Could you check a few things on this model? Use its own coordinates, in mm. A direction names the side the tool comes from. Round coordinates to 2 decimals unless told otherwise and drop trailing zeros. Write each loop counter-clockwise with the first axis right and the second up, starting at its lowest first coordinate (ties: lowest second). Pieces come first, ordered by that corner, then holes. Notation, with made-up numbers: (4, 27) -> (15, 27) arc R15 ccw to (15, 43) -> close; hole circle Ø7 at (58, -22). An arc over 180 degrees is marked (long way). One line per question, with ' | ' between items. Start each with the question number.
1. If I drill on line 1 along Y through (x, z) = (25, 12.5); line 2 along Z through (x, y) = (4, 16); line 3 along X through (y, z) = (55, 9.75), over which ranges is the centre line in solid material (lowest first)? Write a range as [from, to].
2. For pin 1 Ø2 at (x, z) = (1.5, 5.5) entering from +Y; pin 2 Ø12 at (x, y) = (30.5, 23.5) entering from -Z; pin 3 Ø0.6 at (x, z) = (45.5, 10.5) entering from +Y, each with a flat end and sliding along its axis, tell me the tip position at first contact or that it passes through.
3. Imagine slicing it at A-A, the plane y = 9.5. List the corners of the cut face in (x, z) for me, and give its area (3 significant figures).
4. For faces 5 (the flat face through (1, 36.8, 6)), 6 (the flat face through (23, 32, 16.5)), 7 (the flat face through (45, 32, 1)), 8 (the cylindrical face through (46.7, 62.4, 1)), which set-ups out of +Z, -Z, +X, -X, +Y, -Y let a thin tool reach every point of the face, with its end or its side?
5. Imagine slicing it at B-B, the plane z = 7.75. List the corners of the cut face in (x, y) for me.
6. Imagine slicing it at C-C, the plane y = 59.5. List the corners of the cut face in (x, z) for me, and give its area (3 significant figures).
7. Thinking about a two-plate mould opening in X: for faces 1 (the flat face through (23, 32, 0)), 2 (the flat face through (44, 36, 17)), 3 (the flat face through (4, 60, 9)), 4 (the flat face through (46, 30, 17)), which applies, released by +X, released by -X, zero draft, split by the parting line, or undercut?
from build123d import *

# Parameters (mm, degrees)
BOSS_EXTRU_1_DEPTH            = 18.5
ESQUISSE5_W                   = 18.5
ESQUISSE5_H                   = 9.899494937
BOSS_EXTRU_3_DEPTH            = 1.5
CONG_1_R                      = 1.5
ENL_V_MAT_EXTRU_7_DEPTH       = 0.5
ENL_V_START                   = -0.2
ENL_V_MAT_EXTRU_9_DEPTH       = 0.2
ENL_V_START_2                 = -2
ENL_V_MAT_EXTRU_10_DEPTH      = 14.5
ENL_V_MAT_EXTRU_11_DEPTH      = 15.5
ENL_V_MAT_EXTRU_11_DEPTH_BACK = 1
ESQUISSE11_W                  = 2
ESQUISSE11_H                  = 66.45046337
ESQUISSE12_W                  = 2.477505898
ESQUISSE12_H                  = 3.959677151
ENL_V_MAT_EXTRU_12_DEPTH      = 14.5
ENL_V_START_3                 = 3
ESQUISSE13_W                  = 2
ESQUISSE13_H                  = 9
ENL_V_MAT_EXTRU_13_DEPTH      = 2


# Read off the part's stored shape, not the designer's step: Enl_v. mat.-Extru.9
with BuildPart() as part:
    # Esquisse1 → Boss.-Extru.1 (new body)
    with BuildSketch(Plane.XY):
        Polygon((7, 63), (0, 56), (0, 0), (47, 0), (47, 63), align=None)
    extrude(amount=BOSS_EXTRU_1_DEPTH)

    # Esquisse5 → Boss.-Extru.3 (add)
    with BuildSketch(Plane(origin=(-28, 28, 0), x_dir=(0, 0, 1), z_dir=(-0.707106781186549, 0.7071067811865462, 0))):
        with Locations((9.25, 44.547727215)):
            Rectangle(ESQUISSE5_W, ESQUISSE5_H)
    extrude(amount=-BOSS_EXTRU_3_DEPTH)

    # Cong_1
    cong_1_edges = [part.edges().sort_by_distance(p)[0] for p in [
        (0, 0, 9.25),
        (0, 56, 9.25),
        (7, 63, 9.25),
        (47, 63, 9.25),
        (47, 0, 9.25),
    ]]
    fillet(cong_1_edges, radius=CONG_1_R)

    # Esquisse7 → Enl_v. mat.-Extru.7 (cut)
    with BuildSketch(Plane.XY.offset(18.5)):
        with BuildLine():
            add(Edge.make_bspline(
                [(8.741481422, 23.545339958), (8.97426544, 23.884234425), (9.391722632, 24.491982042), (9.801234093, 25.809520444), (9.912339585, 26.761676513), (9.985835627, 27.391525683)],
                knots=[0, 0, 0, 0, 0.299076085, 0.536340353, 1, 1, 1, 1], degree=3))
            add(Edge.make_bspline(
                [(8.800690837, 23.490312703), (8.780021094, 23.50796535), (8.760751258, 23.526652654), (8.741481422, 23.545339958)],
                knots=[0.816445355, 0.816445355, 0.816445355, 0.816445355, 1, 1, 1, 1], degree=3))
            add(Edge.make_bspline(
                [(37.587874359, 43.964061233), (36.322453208, 42.912301808), (33.856892738, 40.863042189), (29.192246001, 38.90002762), (24.068252551, 36.312701669), (18.552137849, 32.455332186), (13.189313268, 28.201783406), (10.124203366, 24.92862823), (8.800690837, 23.490312703)],
                knots=[0, 0, 0, 0, 0.134488449, 0.262038771, 0.413324325, 0.606278792, 0.814215894, 0.974718857, 0.974718857, 0.974718857, 0.974718857], degree=3))
            add(Edge.make_bspline(
                [(9.443588409, 23.726318154), (10.439928849, 24.865322019), (13.17889562, 27.902664607), (18.360152512, 32.08462974), (24.147814444, 36.14388912), (29.439325332, 38.879729859), (34.023974897, 40.940579508), (36.372875034, 42.933300323), (37.587874359, 43.964061233)],
                knots=[0.043476968, 0.043476968, 0.043476968, 0.043476968, 0.167785205, 0.379770977, 0.589080615, 0.748039182, 0.869669971, 1, 1, 1, 1], degree=3))
            add(Edge.make_bspline(
                [(13.209844249, 24.846255718), (12.561216207, 24.741866177), (11.570036096, 24.582346652), (10.21413428, 24.371732671), (9.686497603, 23.950548462), (9.443588409, 23.726318154)],
                knots=[0, 0, 0, 0, 0.449393835, 0.686726756, 0.906490115, 0.906490115, 0.906490115, 0.906490115], degree=3))
            add(Edge.make_bspline(
                [(19.346207327, 27.92037622), (18.649539489, 27.490364128), (17.295751274, 26.654750267), (15.259428846, 25.586185129), (13.871062619, 25.084965025), (13.209844249, 24.846255718)],
                knots=[0, 0, 0, 0, 0.357022344, 0.693777745, 1, 1, 1, 1], degree=3))
            add(Edge.make_bspline(
                [(16.151045098, 28.579318334), (16.706508218, 28.335383374), (17.609553302, 27.93880571), (18.730896282, 27.827227889), (19.225451429, 27.902095693), (19.346207327, 27.92037622)],
                knots=[0, 0, 0, 0, 0.547075637, 0.889409121, 1, 1, 1, 1], degree=3))
            add(Edge.make_bspline(
                [(19.997230823, 28.428298982), (19.766755369, 28.36324029), (19.12544327, 28.182210485), (17.819957633, 28.388483473), (16.776288941, 28.507823681), (16.151045098, 28.579318334)],
                knots=[0, 0, 0, 0, 0.183614026, 0.510917298, 1, 1, 1, 1], degree=3))
            add(Edge.make_bspline(
                [(27.009732384, 33.579925392), (26.292485205, 33.007945409), (24.797708149, 31.815912062), (22.478329122, 30.069627859), (20.822964986, 28.974549539), (19.997230823, 28.428298982)],
                knots=[0, 0, 0, 0, 0.316155138, 0.658882265, 1, 1, 1, 1], degree=3))
            add(Edge.make_bspline(
                [(22.78741232, 33.594631396), (23.47035804, 33.500852352), (24.67880724, 33.334913527), (26.092254902, 33.472354396), (26.813238587, 33.556887188), (27.009732384, 33.579925392)],
                knots=[0, 0, 0, 0, 0.485970736, 0.859908672, 1, 1, 1, 1], degree=3))
            add(Edge.make_bspline(
                [(27.476930827, 33.958322193), (27.261994438, 33.912287048), (26.51014109, 33.751254856), (24.939704804, 33.622032753), (23.589244994, 33.604839722), (22.78741232, 33.594631396)],
                knots=[0, 0, 0, 0, 0.139880518, 0.489305866, 1, 1, 1, 1], degree=3))
            add(Edge.make_bspline(
                [(30.178310683, 36.158566674), (29.975674371, 35.998229226), (29.462468598, 35.592151447), (28.569556831, 34.84941734), (27.869795727, 34.278724604), (27.476930827, 33.958322193)],
                knots=[0, 0, 0, 0, 0.222488299, 0.563483801, 1, 1, 1, 1], degree=3))
            add(Edge.make_bspline(
                [(38.945351674, 45.321538548), (38.420171007, 44.695713388), (36.761155938, 42.718768237), (33.941660103, 39.55384301), (31.404658543, 37.264972007), (30.178310683, 36.158566674)],
                knots=[0, 0, 0, 0, 0.193087, 0.609950563, 1, 1, 1, 1], degree=3))
            add(Edge.make_bspline(
                [(31.252980224, 40.683491056), (32.324827658, 41.14326203), (34.307774375, 41.993850755), (36.826194398, 43.657503938), (38.274775575, 44.794979312), (38.945351674, 45.321538548)],
                knots=[0, 0, 0, 0, 0.387194684, 0.716320628, 1, 1, 1, 1], degree=3))
            add(Edge.make_bspline(
                [(16.565641294, 35.366704907), (18.224543129, 36.00479534), (21.682233863, 37.334783247), (26.615085728, 39.004604912), (29.840038582, 40.172015828), (31.252980224, 40.683491056)],
                knots=[0, 0, 0, 0, 0.341315206, 0.711411851, 1, 1, 1, 1], degree=3))
            add(Edge.make_bspline(
                [(17.320172435, 32.538627168), (17.095643767, 33.034221194), (16.740497225, 33.818123337), (16.398777614, 34.815395743), (16.52931247, 35.246676309), (16.565641294, 35.366704907)],
                knots=[0, 0, 0, 0, 0.553685075, 0.875787227, 1, 1, 1, 1], degree=3))
            add(Edge.make_bspline(
                [(15.932717497, 35.050525816), (15.968390486, 34.968733309), (16.124488937, 34.610824317), (16.392954493, 33.675509429), (16.95320176, 32.988577964), (17.320172435, 32.538627168)],
                knots=[0, 0, 0, 0, 0.092717793, 0.405716039, 1, 1, 1, 1], degree=3))
            add(Edge.make_bspline(
                [(14.793567783, 34.518281585), (14.908073567, 34.57528331), (15.147913789, 34.694677334), (15.52805859, 34.871411668), (15.794398468, 34.989301673), (15.932717497, 35.050525816)],
                knots=[0, 0, 0, 0, 0.305139846, 0.639136348, 1, 1, 1, 1], degree=3))
            add(Edge.make_bspline(
                [(9.985835627, 27.391525683), (10.083402404, 28.278864149), (10.285137329, 30.113578429), (11.930749087, 32.794310056), (13.772036135, 33.90312161), (14.793567783, 34.518281585)],
                knots=[0, 0, 0, 0, 0.294280708, 0.608472459, 1, 1, 1, 1], degree=3))
        make_face()
    extrude(amount=-ENL_V_MAT_EXTRU_7_DEPTH, mode=Mode.SUBTRACT)

    # Enl_v. mat.-Extru.9 outline → Enl_v. mat.-Extru.9 (cut)
    with BuildSketch(Plane.XY.offset(18.5).offset(ENL_V_START)):
        with BuildLine():
            add(Edge.make_bspline(
                [(9.219208695, 23.519291104), (9.176868463, 23.503048303), (9.073549799, 23.463412607), (8.952624187, 23.520506831), (8.892403529, 23.568918107), (8.882487225, 23.577386959)],
                knots=[0, 0, 0, 0, 0.298493917, 0.728385063, 0.816445357, 0.816445357, 0.816445357, 0.816445357], degree=3))
            add(Edge.make_bspline(
                [(8.882487225, 23.577386959), (8.674018117, 23.350835), (8.465840191, 23.123974501), (8.257662264, 22.897114002)],
                knots=[0.974718857, 0.974718857, 0.974718857, 0.974718857, 1, 1, 1, 1], degree=3))
            add(Edge.make_bspline(
                [(8.257662264, 22.897114002), (8.120380319, 22.724431783), (7.726303318, 22.228735927), (7.172014223, 21.551305412), (6.767070551, 21.036911066), (6.617377175, 20.846757641)],
                knots=[0, 0, 0, 0, 0.25204317, 0.723506773, 1, 1, 1, 1], degree=3))
            add(Edge.make_bspline(
                [(6.617377175, 20.846757641), (6.67105197, 20.876575617), (6.846524977, 20.974056193), (7.146714282, 21.163568152), (7.411642244, 21.289656477), (7.550642829, 21.355811634)],
                knots=[0, 0, 0, 0, 0.173191566, 0.566195825, 1, 1, 1, 1], degree=3))
            add(Edge.make_bspline(
                [(7.550642829, 21.355811634), (7.594875595, 21.408819409), (7.758493986, 21.604896833), (8.073049619, 22.022428419), (8.331605023, 22.394899892), (8.483908483, 22.614306228)],
                knots=[0, 0, 0, 0, 0.132137543, 0.488780926, 1, 1, 1, 1], degree=3))
            add(Edge.make_bspline(
                [(8.483908483, 22.614306228), (8.812805546, 22.994323471), (9.141702609, 23.374340714), (9.472283444, 23.752655313)],
                knots=[0, 0, 0, 0, 0.041267951, 0.041267951, 0.041267951, 0.041267951], degree=3))
            add(Edge.make_bspline(
                [(9.472283444, 23.752655313), (9.46270077, 23.743911905), (9.453136271, 23.735131818), (9.443588409, 23.726318154)],
                knots=[0.897852031, 0.897852031, 0.897852031, 0.897852031, 0.906490115, 0.906490115, 0.906490115, 0.906490115], degree=3))
            add(Edge.make_bspline(
                [(9.443588409, 23.726318154), (9.460918461, 23.746129651), (9.478253382, 23.765936224), (9.495593415, 23.785737628)],
                knots=[0.043476968, 0.043476968, 0.043476968, 0.043476968, 0.045639149, 0.045639149, 0.045639149, 0.045639149], degree=3))
            add(Edge.make_bspline(
                [(9.495593415, 23.785737628), (9.40250572, 23.698858445), (9.310857207, 23.609074775), (9.219208695, 23.519291104)],
                knots=[0.915490159, 0.915490159, 0.915490159, 0.915490159, 1, 1, 1, 1], degree=3))
        make_face()
    extrude(amount=ENL_V_MAT_EXTRU_9_DEPTH, mode=Mode.SUBTRACT)

    # Esquisse10 → Enl_v. mat.-Extru.10 (cut)
    with BuildSketch(Plane(origin=(0, 0, 0), x_dir=(-1, 0, 0), z_dir=(0, 0, -1)).offset(ENL_V_START_2)):
        Polygon((-47.600891072, 61), (-7.828427125, 61), (-2, 55.171572875), (-2, 2), (-47.600891072, 2), align=None)
    extrude(amount=-ENL_V_MAT_EXTRU_10_DEPTH, mode=Mode.SUBTRACT)

    # Esquisse11 → Enl_v. mat.-Extru.11 (cut, two sides: drawn at the far end of the back side and taken through both)
    with BuildSketch(Plane.XY.offset(2).offset(-ENL_V_MAT_EXTRU_11_DEPTH_BACK)):
        with Locations((45, 34.225231685)):
            Rectangle(ESQUISSE11_W, ESQUISSE11_H)
    extrude(amount=ENL_V_MAT_EXTRU_11_DEPTH + ENL_V_MAT_EXTRU_11_DEPTH_BACK, mode=Mode.SUBTRACT)

    # Esquisse12 → Enl_v. mat.-Extru.12 (cut)
    with BuildSketch(Plane.XY.offset(2)):
        with Locations((47.238752949, 61.767431922)):
            Rectangle(ESQUISSE12_W, ESQUISSE12_H)
    extrude(amount=ENL_V_MAT_EXTRU_12_DEPTH, mode=Mode.SUBTRACT)

    # Esquisse13 → Enl_v. mat.-Extru.13 (cut)
    with BuildSketch(Plane.XY.offset(2).offset(ENL_V_START_3)):
        with Locations((1, 41.3)):
            Rectangle(ESQUISSE13_W, ESQUISSE13_H)
    extrude(amount=ENL_V_MAT_EXTRU_13_DEPTH, mode=Mode.SUBTRACT)


solid = part.part
Geometry results:
1) line 1: y = [0, 2], [61, 63] | line 2: z = [0, 2], [16.5, 18.5] | line 3: x = [0, 2]
2) pin 1: stops at y = 58.5 | pin 2: stops at z = 0 | pin 3: stops at y = 1
3) outline: (0, 0) -> (47, 0) -> (47, 2) -> (46, 2) -> (46, 1) -> (44, 1) -> (44, 2) -> (2, 2) -> (2, 16.5) -> (44, 16.5) -> (44, 17.5) -> (46, 17.5) -> (46, 16.5) -> (47, 16.5) -> (47, 18.5) -> (0, 18.5) -> close | area: 213 mm2
4) face 5: +X, -X | face 6: +X | face 7: +Y | face 8: +Z, -Z, +X, +Y
5) outline: (0, 1.5) arc R1.5 ccw to (1.5, 0) -> (45.5, 0) arc R1.5 ccw to (47, 1.5) -> (47, 2) -> (46, 2) -> (46, 1) -> (44, 1) -> (44, 2) -> (2, 2) -> (2, 55.17) -> (7.83, 61) -> (44, 61) -> (44, 63) -> (7.62, 63) arc R1.5 ccw to (6.56, 62.56) -> (0.44, 56.44) arc R1.5 ccw to (0, 55.38) -> close
6) outline: (3.5, 0) -> (47, 0) -> (47, 2) -> (46, 2) -> (46, 1) -> (44, 1) -> (44, 2) -> (6.33, 2) -> (6.33, 16.5) -> (44, 16.5) -> (44, 17.5) -> (46, 17.5) -> (46, 16.5) -> (47, 16.5) -> (47, 18.5) -> (3.5, 18.5) -> close | area: 211 mm2
7) face 1: zero draft | face 2: undercut | face 3: released by -X | face 4: undercut
